Design review of the part built by this model. Coordinates are the model's own, in mm. A direction names the side the tool comes from. Give positions to 0.01 mm unless a question says otherwise; leave off trailing zeros. Loops run counter-clockwise (first coordinate to the right, second up) from the corner with the lowest first, then second, coordinate; pieces in that order, holes last. Notation, with made-up numbers: (38, -11.75) -> (90, -11.75) arc R19 ccw to (90, 20.25) -> close; hole circle Ø8 at (76, 2.5). An arc over 180 degrees is marked (long way). Use CSV: the item, a comma, the result in double quotes. Start each with the question number.
Item 1: We need section D-D (z = -6.5). State the section outline as (x, y) points (3 decimals).
Item 2: We need section C-C (x = 0). State the section outline as (y, z) points (3 decimals).
Item 3: The part is to be moulded in two halves that separate along X. For faces 1 (the face through (14.55, 0.96, 14.26)), 2 (the face through (0, 0, 0)), 3 (the face through (14.55, 0.96, -13.24)), 4 (the face through (19, 1, 0)), say which applies: +X half, -X half, draft (parallel to the pull), parting line (faces both ways), or undercut.
Item 4: We need section B-B (z = 13.75). State the section outline as (x, y) points, plus the area to 3 significant figures.
Item 5: Clearance check with flat-ended pins moving along their axes: pin 1 (4 mm diameter, centred on x = -12.5, z = -7, fed in from +Y); pin 2 (2 mm diameter, centred on y = 5, z = 3.5, fed in from +X) (3 decimals); pin 3 (8 mm diameter, centred on x = -14, y = 19, fed in from -Z); pin 4 (2 mm diameter, centred on y = 4.5, z = 0.5, fed in from -X) (3 decimals). State where each tip first meets the part, or that it passes through.
Item 6: Wall thickness on line 1 along X through (y, z) = (0.9, 13.75); line 2 along Y through (x, z) = (-12.5, 16.5); line 3 along Z through (x, y) = (-6.5, 7.75) (3 decimals): over which ranges is each line inside the solid? List them lowest first. Write a range as from..to.
Item 7: We need section A-A (x = -13.75). State the section outline as (y, z) points, plus the area to 3 significant figures.
Item 8: For faces 5 (the face through (0, 5, 8.085)), 6 (the face through (0, 5, -8.085)), 7 (the face through (0.33, 18.024, -7.493)), list the 3-axis set-ups (+Z, -Z, +X, -X, +Y, -Y) from which the entire face can be reached by the end or side of a thin tool; tool diameter is ignored.
from build123d import *

# Parameters (mm, degrees)
SKETCH1_W           = 38
SKETCH1_H           = 38
BOSS_EXTRUDE1_DEPTH = 1.9
SKETCH2_W           = 16.17
SKETCH2_H           = 16.17
BOSS_EXTRUDE2_DEPTH = 7.25
SKETCH4_R           = 7.5
BOSS_EXTRUDE3_DEPTH = 18
SKETCH5_R           = 0.95
CUT_EXTRUDE1_DEPTH  = 18


with BuildPart() as part:
    # Sketch1 → Boss-Extrude1 (new body)
    with BuildSketch(Plane(origin=(0, 0, 0), x_dir=(1, 0, 0), z_dir=(0, 1, 0))):
        Rectangle(SKETCH1_W, SKETCH1_H)
    extrude(amount=BOSS_EXTRUDE1_DEPTH)

    # Sketch2 → Boss-Extrude2 (add)
    with BuildSketch(Plane(origin=(0, 1.9, 0), x_dir=(1, 0, 0), z_dir=(0, 1, 0))):
        Rectangle(SKETCH2_W, SKETCH2_H)
    extrude(amount=BOSS_EXTRUDE2_DEPTH)

    # Sketch4 → Boss-Extrude3 (add)
    with BuildSketch(Plane(origin=(0, 9.15, 0), x_dir=(1, 0, 0), z_dir=(0, 1, 0))):
        with Locations(Location((0, 0, 0), (0, 0, 270))):
            Circle(SKETCH4_R)
    extrude(amount=BOSS_EXTRUDE3_DEPTH)

    # Sketch5 → Cut-Extrude1 (cut)
    with BuildSketch(Plane(origin=(0, 1.9, 0), x_dir=(1, 0, 0), z_dir=(0, 1, 0))):
        with Locations(Location((-13.75, 13.75, 0), (0, 0, 270))):
            Circle(SKETCH5_R)
        with Locations(Location((13.75, 13.75, 0), (0, 0, 270))):
            Circle(SKETCH5_R)
        with Locations(Location((13.75, -13.75, 0), (0, 0, 270))):
            Circle(SKETCH5_R)
        with Locations(Location((-13.75, -13.75, 0), (0, 0, 270))):
            Circle(SKETCH5_R)
    extrude(amount=-CUT_EXTRUDE1_DEPTH, mode=Mode.SUBTRACT)


solid = part.part
Results found:
1,outline,"(-19, 0) -> (19, 0) -> (19, 1.9) -> (8.085, 1.9) -> (8.085, 9.15) -> (3.742, 9.15) -> (3.742, 27.15) -> (-3.742, 27.15) -> (-3.742, 9.15) -> (-8.085, 9.15) -> (-8.085, 1.9) -> (-19, 1.9) -> close"
2,outline,"(0, -19) -> (1.9, -19) -> (1.9, -8.085) -> (9.15, -8.085) -> (9.15, -7.5) -> (27.15, -7.5) -> (27.15, 7.5) -> (9.15, 7.5) -> (9.15, 8.085) -> (1.9, 8.085) -> (1.9, 19) -> (0, 19) -> close"
3,face 1,"undercut"
3,face 2,"draft"
3,face 3,"undercut"
3,face 4,"+X half"
4,outline,"(-19, 0) -> (-14.7, 0) -> (-14.7, 1.9) -> (-19, 1.9) -> close; (-12.8, 0) -> (12.8, 0) -> (12.8, 1.9) -> (-12.8, 1.9) -> close; (14.7, 0) -> (19, 0) -> (19, 1.9) -> (14.7, 1.9) -> close"
4,area,"65.0 mm²"
5,pin 1,"y = 1.9"
5,pin 2,"x = 8.085"
5,pin 3,"through"
5,pin 4,"x = -8.085"
6,line 1,"-19..-14.7, -12.8..12.8, 14.7..19"
6,line 2,"0..1.9"
6,line 3,"-8.085..8.085"
7,outline,"(0, -19) -> (1.9, -19) -> (1.9, -14.7) -> (0, -14.7) -> close; (0, -12.8) -> (1.9, -12.8) -> (1.9, 12.8) -> (0, 12.8) -> close; (0, 14.7) -> (1.9, 14.7) -> (1.9, 19) -> (0, 19) -> close"
7,area,"65.0 mm²"
8,face 5,"+Z, +X, -X, +Y"
8,face 6,"-Z, +X, -X, +Y"
8,face 7,"+Y"
